Autodesk Inventor part; units mm, degrees
ref_plane "YZ Plane" through (0, 0, 0) normal (1, 0, 0) x (0, 1, 0)
ref_plane "XZ Plane" through (0, 0, 0) normal (0, 1, 0) x (-1, 0, 0)
ref_plane "XY Plane" through (0, 0, 0) normal (0, 0, 1) x (1, 0, 0)
sketch "Sketch1" plane through (0, 0, 0) normal (0, 0, 1) x (1, 0, 0)
  line L0 (3.9669, 12.6467) -> (5.1169, 12.6467)
  line L1 (5.1169, 12.6467) -> (5.1169, 1.1467)
  line L2 (5.1169, 1.1467) -> (16.6169, 1.1467)
  line L3 (16.6169, 1.1467) -> (16.6169, -1.1533)
  line L4 (16.6169, -1.1533) -> (5.1169, -1.1533)
  line L5 (5.1169, -1.1533) -> (5.1169, -12.6533)
  line L6 (5.1169, -12.6533) -> (3.9669, -12.6533)
  line L7 (3.9669, 12.6467) -> (2.8169, 12.6467)
  line L8 (2.8169, 12.6467) -> (2.8169, 1.1467)
  line L9 (2.8169, 1.1467) -> (-8.6831, 1.1467)
  line L10 (-8.6831, 1.1467) -> (-8.6831, -1.1533)
  line L11 (-8.6831, -1.1533) -> (2.8169, -1.1533)
  line L12 (2.8169, -1.1533) -> (2.8169, -12.6533)
  line L13 (2.8169, -12.6533) -> (3.9669, -12.6533)
  point P0 (0, 0)
  dimension "d0" = 1.15
  dimension "d1" = 2.3
  dimension "d2" = 11.5
  dimension "d3" = 11.5
  dimension "d4" = 11.5
  dimension "d5" = 11.5
  dimension "d6" = 1.15
extrude "Extrusion1" add sketch "Sketch1" along normal blind 140
ref_plane "Work Plane1" through (3.9669, 1.1467, 0) normal (-1, 0, 0) x (0, 0, 1)
sketch "Sketch4" plane through (3.9669, 1.1467, 0) normal (-1, 0, 0) x (0, 0, 1)
  line L0 (3.9669, 12.6467) -> (5.1169, 12.6467)
  line L1 (5.1169, 12.6467) -> (5.1169, 1.1467)
  line L2 (5.1169, 1.1467) -> (16.6169, 1.1467)
  line L3 (16.6169, 1.1467) -> (16.6169, -1.1533)
  line L4 (16.6169, -1.1533) -> (5.1169, -1.1533)
  line L5 (5.1169, -1.1533) -> (5.1169, -12.6533)
  line L6 (5.1169, -12.6533) -> (3.9669, -12.6533)
  line L7 (2.8169, 12.6467) -> (2.8169, 1.1467)
  line L8 (2.8169, 1.1467) -> (-8.6831, 1.1467)
  line L9 (-8.6831, 1.1467) -> (-8.6831, -1.1533)
  line L10 (-8.6831, -1.1533) -> (2.8169, -1.1533)
  line L11 (2.8169, -1.1533) -> (2.8169, -12.6533)
  line L12 (2.8169, -12.6533) -> (3.9669, -12.6533)
  line L13 (3.9669, 12.6467) -> (2.8169, 12.6467)
  line L14 (140, -13.8) -> (140, 11.5)
  line L15 (140, -13.6427) -> (140, -13.8)
  line L16 (140, -2.3) -> (140, -13.6427)
  line L17 (140, 0) -> (140, -2.3)
  line L18 (140, 11.3427) -> (140, 0)
  line L19 (140, 11.5) -> (140, 11.3427)
  line L20 (154, -1.15) -> (140, 12.35)
  line L21 (140, 11.3427) -> (140, 0)
  line L22 (154, -1.15) -> (140, -1.15)
  line L23 (140, 12.35) -> (140, -1.15)
  line L24 (154.6806, -1.15) -> (155.8888, -1.15)
  point P0 (0, -1.1467)
  point P1 (0, 0)
  point P2 (154, -1.15)
  dimension "d13" = 1.15
  dimension "d14" = 2.3
  dimension "d15" = 11.5
  dimension "d16" = 11.5
  dimension "d17" = 11.5
  dimension "d18" = 11.5
  dimension "d19" = 1.15
revolve "Revolution2" add sketch "Sketch4" angle 360 about axis through (3.9669, -0.0033, 154.6806) along (0, 0, 1) contours L14 L23 L20 L22
sketch "Sketch5" plane through (0, 0, 0) normal (0, 0, -1) x (-1, 0, 0)
  circle A0 centre (-3.9669, -0.0033) radius 13.5
  circle A1 centre (-3.9669, -0.0033) radius 15.45
  point P0 (0, 0)
  dimension "d21" = 30.9
extrude "Extrusion2" add sketch "Sketch5" along normal blind 1.87 contours A0 | A1
sketch "Sketch6" plane through (3.9669, 1.1467, 0) normal (-1, 0, 0) x (0, 0, 1)
  line L0 (0, 11.5) -> (0, 0)
  line L1 (0, 11.5) -> (140, 11.5)
  line L2 (0, -1.1467) -> (5.329, -1.1467)
  line L3 (0, 14.3) -> (-1.87, 14.3)
  line L4 (0, 14.3) -> (0, 7.3)
  line L5 (0, 0) -> (0, 11.5)
  line L6 (0, 14.3) -> (18, 14.3)
  line L7 (18, 14.3) -> (0, 5.75)
  point P0 (0, 7.85)
  point P1 (12, 11.5)
  dimension "d27" = 7
revolve "Revolution3" cut sketch "Sketch6" angle 360 about axis through (3.9669, 0, 0) along (0, 0, 1)
properties part number "syringe inner"
Verification items for the finished model (mm, model axes). A direction names the side the tool comes from. Coordinates: 2 decimals unless noted, no trailing zeros. Order: outer loops, then holes, each group sorted by start corner. A loop starts at its lowest first (then second) coordinate and runs counter-clockwise, first axis right, second up. Notation, with made-up numbers: (28.5, 6.5) - (86.5, 6.5) arc R17 cw to (86.5, 24.5) - close; hole circle Ø11 at (-14, -13.5). An arc over 180 degrees is marked (long way). Return JSON: item names as keys, results as strings.
(1) Thickness scan on line 1 along Y through (x, z) = (12.5, 84); line 2 along Z through (x, y) = (16, 8.5); line 3 along X through (y, z) = (-5.5, 27). Record the ranges inside material, lowest first.
Filled sheet:
{"line 1": "y = -1.15 to 1.15", "line 2": "z = -1.87 to 0", "line 3": "x = 2.82 to 5.12"}
(2) Mould release check, pull along Z, two halves, no side actions. Record for faces 6 (the flat face through (11, -1.153, 69)), 7 (the cylindrical face through (-10.77, -4.64, -0.92)), 8 (the conical face through (5.122, 3.664, 150.013)): pulls with the +Z half, pulls with the -Z half, needs draft (parallel to the pull), parting line crosses it, or undercut.
Filled sheet:
{"face 6": "undercut", "face 7": "needs draft", "face 8": "pulls with the +Z half"}
(3) Section check A-A, the plane z = 21. Record the cut outline in (x, y), and give its area (3 significant figures).
Filled sheet:
{"outline": "(-8.68, -1.15) - (2.82, -1.15) - (2.82, -12.65) - (5.12, -12.65) - (5.12, -1.15) - (16.62, -1.15) - (16.62, 1.15) - (5.12, 1.15) - (5.12, 12.65) - (2.82, 12.65) - (2.82, 1.15) - (-8.68, 1.15) - close", "area": "111 mm^2"}
(4) Go/stop test with flat-tipped pins: pin 1 (9 mm diameter, centred on x = 13, z = 75.5, fed in from -Y); pin 2 (12.5 mm diameter, centred on x = 8.5, z = 77, fed in from +Y); pin 3 (5 mm diameter, centred on x = 0.5, z = 104, fed in from -Y). Record where each tip stops, or that it passes through.
Filled sheet:
{"pin 1": "stops at y = -1.15", "pin 2": "stops at y = 12.65", "pin 3": "stops at y = -12.65"}
(5) Access from +Z, -Z, +X, -X, +Y, -Y to the whole of each face (thin tool, end or side, straight path). Record for faces 1 (the flat face through (2.817, 7, 69)), 2 (the flat face through (5.117, 7, 69)), 3 (the flat face through (5.117, -7, 69)), 4 (the flat face through (2.817, -7, 69)), 5 (the flat face through (7, 3, 140)).
Filled sheet:
{"face 1": "-X, +Y", "face 2": "+X, +Y", "face 3": "+X, -Y", "face 4": "-X, -Y", "face 5": "none"}
